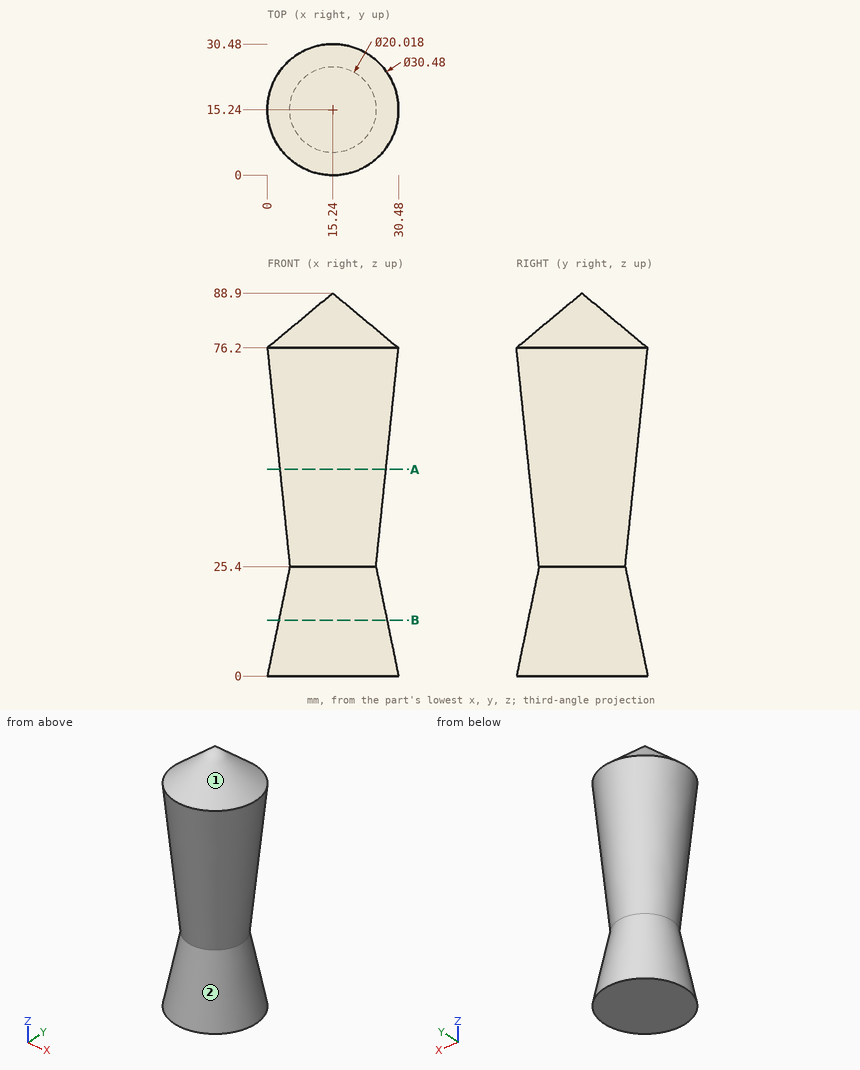
Geometry: see drawing. Coordinates: mm, zero at the bounding-box minimum. A direction names the side the tool comes from. Give positions to 0.01 mm unless a question says otherwise; leave off trailing zeros. Order: outer loops, then holes, each group sorted by start corner. A loop starts at its lowest first (then second) coordinate and runs counter-clockwise, first axis right, second up. Notation, with made-up numbers: (24, -18) - (76, -18) arc R28 ccw to (76, 5) - close; hole circle Ø6 at (52.5, 89). An arc over 180 degrees is marked (long way). One line per item, written item: value.
1. Line query: probe 1 along Z at (x, y) = (10.5, 9.5); probe 2 along X at (y, z) = (5.5, 62.5); probe 3 along X at (y, z) = (15, 29). Output: solid intervals per line, ascending.
Determined:
probe 1: 0 to 82.7
probe 2: 5.42 to 25.06
probe 3: 4.86 to 25.62
2. Reachability of the marked faces 1 and 2 from +Z, -Z, +X, -X, +Y, -Y: full face, straight path, thin tool, end or side. Return the list, or none.
Determined:
face 1: +Z
face 2: none
3. Cut plane A-A, the plane z = 48. Output: boundary loops of the cut face in (x, y), and give its area (3 significant figures).
Determined:
outline: circle Ø24.67 at (15.24, 15.24)
area: 478 mm2
4. Cut plane B-B, the plane z = 13. Output: boundary loops of the cut face in (x, y).
Determined:
outline: circle Ø25.13 at (15.24, 15.24)
5. Pin query (flat end, axial travel): pin 1 Ø10 at (x, z) = (27.5, 64) entering from +Y; pin 2 Ø12 at (x, z) = (20.5, 24) entering from -Y; pin 3 Ø8 at (x, z) = (16, 38) entering from +Y. Return the tip coordinate at first contact, or that it passes through.
Determined:
pin 1: y = 27.25
pin 2: y = 4.08
pin 3: y = 26.95
